Autodesk Inventor part; units mm, degrees
ref_plane "YZ Plane" through (0, 0, 0) normal (1, 0, 0) x (0, 1, 0)
ref_plane "XZ Plane" through (0, 0, 0) normal (0, 1, 0) x (-1, 0, 0)
ref_plane "XY Plane" through (0, 0, 0) normal (0, 0, 1) x (1, 0, 0)
sketch "Skizze1" plane through (0, 0, 0) normal (0, 0, 1) x (1, 0, 0)
  line L0 (0, -42.3366) -> (0, 42.3366) construction
  line L1 (-38.4382, 0) -> (56.3005, 0) construction
  line L2 (0, 0) -> (30.2404, 30.2404) construction
  line L3 (0, 0) -> (42.7664, 0) construction
  line L4 (0, 24.9041) -> (16.9, 24.9041)
  line L5 (16.9, 24.9041) -> (16.9, 21.2841)
  line L6 (16.9, 21.2841) -> (19.092, 19.092)
  line L7 (24.9041, 0) -> (24.9041, 16.9)
  line L8 (24.9041, 16.9) -> (21.2841, 16.9)
  line L9 (21.2841, 16.9) -> (19.092, 19.092)
  line L10 (0, 24.9041) -> (-16.9, 24.9041)
  line L11 (-16.9, 24.9041) -> (-16.9, 21.2841)
  line L12 (-16.9, 21.2841) -> (-19.092, 19.092)
  line L13 (-24.9041, 0) -> (-24.9041, 16.9)
  line L14 (-24.9041, 16.9) -> (-21.2841, 16.9)
  line L15 (-21.2841, 16.9) -> (-19.092, 19.092)
  line L16 (0, 0) -> (30.2404, -30.2404) construction
  line L17 (0, -24.9041) -> (16.9, -24.9041)
  line L18 (16.9, -24.9041) -> (16.9, -21.2841)
  line L19 (16.9, -21.2841) -> (19.092, -19.092)
  line L20 (24.9041, 0) -> (24.9041, -16.9)
  line L21 (24.9041, -16.9) -> (21.2841, -16.9)
  line L22 (21.2841, -16.9) -> (19.092, -19.092)
  line L23 (0, -24.9041) -> (-16.9, -24.9041)
  line L24 (-16.9, -24.9041) -> (-16.9, -21.2841)
  line L25 (-16.9, -21.2841) -> (-19.092, -19.092)
  line L26 (-24.9041, 0) -> (-24.9041, -16.9)
  line L27 (-24.9041, -16.9) -> (-21.2841, -16.9)
  line L28 (-21.2841, -16.9) -> (-19.092, -19.092)
  circle A0 centre (0, 0) radius 10
  dimension "d0" = 45
  dimension "d1" = 16.9
  dimension "d2" = 3.1
  dimension "d3" = 3.62
  dimension "d4" = 20
extrude "Extrusion1" add sketch "Skizze1" along normal blind 2.5
sketch "Skizze2" plane through (0, 0, 2.5) normal (0, 0, 1) x (1, 0, 0)
  line L0 (17.3243, 16.97) -> (5, 16.97) construction
  line L1 (17.3243, 16.97) -> (17.3243, 14.47) construction
  line L2 (5, 14.47) -> (17.3243, 14.47) construction
  line L3 (5, 16.97) -> (5, 14.47) construction
  line L4 (-5, 16.97) -> (-17.3243, 16.97) construction
  line L5 (-5, 16.97) -> (-5, 14.47) construction
  line L6 (-17.3243, 14.47) -> (-5, 14.47) construction
  line L7 (-17.3243, 16.97) -> (-17.3243, 14.47) construction
  circle A0 centre (0, 0) radius 10 construction
  line L8 (16.9, 24.9041) -> (-16.9, 24.9041) construction
  line L9 (-16.9, 24.9041) -> (-16.9, 21.2841) construction
  line L10 (-16.9, 21.2841) -> (-21.2841, 16.9) construction
  line L11 (-21.2841, 16.9) -> (-24.9041, 16.9) construction
  line L12 (-24.9041, 16.9) -> (-24.9041, -16.9) construction
  line L13 (-24.9041, -16.9) -> (-21.2841, -16.9) construction
  line L14 (-21.2841, -16.9) -> (-16.9, -21.2841) construction
  line L15 (-16.9, -21.2841) -> (-16.9, -24.9041) construction
  line L16 (-16.9, -24.9041) -> (16.9, -24.9041) construction
  line L17 (16.9, -24.9041) -> (16.9, -21.2841) construction
  line L18 (16.9, -21.2841) -> (21.2841, -16.9) construction
  line L19 (21.2841, -16.9) -> (24.9041, -16.9) construction
  line L20 (24.9041, -16.9) -> (24.9041, 16.9) construction
  line L21 (24.9041, 16.9) -> (21.2841, 16.9) construction
  line L22 (21.2841, 16.9) -> (16.9, 21.2841) construction
  line L23 (16.9, 21.2841) -> (16.9, 24.9041) construction
  line L24 (-5, 14.47) -> (5, 14.47) construction
  line L25 (5, 14.47) -> (5, 24.9041) construction
  line L26 (5, 24.9041) -> (-5, 24.9041) construction
  line L27 (-5, 24.9041) -> (-5, 14.47) construction
  line L28 (-16.9, 21.2841) -> (-21.2841, 16.9) construction
  line L29 (-16.9, 21.2841) -> (-24.9041, 21.2841) construction
  line L30 (-24.9041, 21.2841) -> (-24.9041, 14.47) construction
  line L31 (-24.9041, 14.47) -> (-16.9, 14.47) construction
  line L32 (-16.9, 14.47) -> (-16.9, 21.2841) construction
  line L33 (0, -34.8857) -> (0, 34.9857) construction
  line L34 (-24.9041, 16.9) -> (-24.9041, -16.9) construction
  line L35 (17.3243, 16.97) -> (17.3243, 14.47) construction
  line L36 (16.9, 21.2841) -> (21.2841, 16.9) construction
  line L37 (21.2841, 16.9) -> (24.9041, 16.9) construction
  line L38 (16.9, 21.2841) -> (21.2841, 16.9) construction
  line L39 (16.9, 21.2841) -> (24.9041, 21.2841) construction
  line L40 (24.9041, 21.2841) -> (24.9041, 14.47) construction
  line L41 (24.9041, 14.47) -> (16.9, 14.47) construction
  line L42 (16.9, 14.47) -> (16.9, 21.2841) construction
  line L43 (16.8, 14.37) -> (25.0041, 14.37)
  line L44 (25.0041, 14.37) -> (25.0041, 21.3841)
  line L45 (25.0041, 21.3841) -> (16.8, 21.3841)
  line L46 (16.8, 21.3841) -> (16.8, 14.37)
  line L47 (-16.8, 14.37) -> (-25.0041, 14.37)
  line L48 (-25.0041, 14.37) -> (-25.0041, 21.3841)
  line L49 (-25.0041, 21.3841) -> (-16.8, 21.3841)
  line L50 (-16.8, 21.3841) -> (-16.8, 14.37)
  line L51 (16.9, 24.9041) -> (-16.9, 24.9041) construction
  line L52 (-5, 14.47) -> (5, 14.47) construction
  line L53 (5, 14.47) -> (5, 24.9041) construction
  line L54 (5, 24.9041) -> (-5, 24.9041) construction
  line L55 (-5, 24.9041) -> (-5, 14.47) construction
  line L56 (5.1, 25.0041) -> (5.1, 14.37)
  line L57 (5.1, 14.37) -> (-5.1, 14.37)
  line L58 (-5.1, 14.37) -> (-5.1, 25.0041)
  line L59 (-5.1, 25.0041) -> (5.1, 25.0041)
  dimension "d8" = 0.1
  dimension "d9" = 0.1
  dimension "d15" = 10
  dimension "d16" = 0.1
extrude "Extrusion2" cut sketch "Skizze2" against normal through all
sketch "Skizze3" plane through (0, 0, 2.5) normal (0, 0, 1) x (1, 0, 0)
  line L0 (16.8, 21.3841) -> (16.9, 21.3841) construction
  line L1 (16.9, 21.3841) -> (16.9, 24.9041) construction
  line L2 (-5.1, 24.9041) -> (-16.9, 24.9041) construction
  line L3 (16.9, 24.9041) -> (5.1, 24.9041) construction
  line L4 (-16.9, 24.9041) -> (-16.9, 21.3841) construction
  line L5 (-16.9, 21.3841) -> (-16.8, 21.3841) construction
  line L6 (-16.8, 21.3841) -> (-16.8, 14.37) construction
  line L7 (-16.8, 14.37) -> (-24.9041, 14.37) construction
  line L8 (-24.9041, 14.37) -> (-24.9041, -16.9) construction
  line L9 (-24.9041, -16.9) -> (-21.2841, -16.9)
  line L10 (-21.2841, -16.9) -> (-16.9, -21.2841)
  line L11 (-16.9, -21.2841) -> (-16.9, -24.9041)
  line L12 (-16.9, -24.9041) -> (16.9, -24.9041) construction
  line L13 (16.9, -24.9041) -> (16.9, -21.2841)
  line L14 (16.9, -21.2841) -> (21.2841, -16.9)
  line L15 (21.2841, -16.9) -> (24.9041, -16.9)
  line L16 (24.9041, -16.9) -> (24.9041, 14.37) construction
  line L17 (24.9041, 14.37) -> (16.8, 14.37) construction
  line L18 (16.8, 14.37) -> (16.8, 21.3841) construction
  circle A0 centre (0, 0) radius 10 construction
  line L19 (24.8041, -16.8) -> (21.2426, -16.8)
  line L20 (21.2426, -16.8) -> (16.8, -21.2426)
  line L21 (16.8, -21.2426) -> (16.8, -24.8041)
  line L22 (16.8, -24.8041) -> (-16.8, -24.8041) construction
  line L23 (-16.8, -24.8041) -> (-16.8, -21.2426)
  line L24 (-16.8, -21.2426) -> (-21.2426, -16.8)
  line L25 (-21.2426, -16.8) -> (-24.8041, -16.8)
  line L26 (-24.8041, -16.8) -> (-24.8041, 14.27) construction
  line L27 (-24.8041, 14.27) -> (-16.7, 14.27) construction
  line L28 (-16.7, 14.27) -> (-16.7, 21.4841) construction
  line L29 (-16.7, 21.4841) -> (-16.8, 21.4841) construction
  line L30 (-16.8, 21.4841) -> (-16.8, 24.8041) construction
  line L31 (-16.8, 24.8041) -> (-2.7, 24.8041) construction
  line L32 (-2.7, 24.8041) -> (-2.7, 14.27) construction
  line L33 (-2.7, 14.27) -> (2.7, 14.27) construction
  line L34 (2.7, 14.27) -> (2.7, 24.8041) construction
  line L35 (2.7, 24.8041) -> (16.8, 24.8041) construction
  line L36 (16.8, 24.8041) -> (16.8, 21.4841) construction
  line L37 (16.8, 21.4841) -> (16.7, 21.4841) construction
  line L38 (16.7, 21.4841) -> (16.7, 14.27) construction
  line L39 (16.7, 14.27) -> (24.8041, 14.27) construction
  line L40 (24.8041, 14.27) -> (24.8041, -16.8) construction
  line L41 (-24.8041, -16.8) -> (-24.8041, -16.9)
  line L42 (-16.8, -24.8041) -> (-16.9, -24.8041)
  line L43 (16.8, -24.8041) -> (16.9, -24.8041)
  line L44 (24.8041, -16.8) -> (24.8041, -16.9)
  line L45 (5.1, 24.9041) -> (5.1, 14.37)
  line L46 (5.1, 14.37) -> (-5.1, 14.37)
  line L47 (-5.1, 14.37) -> (-5.1, 24.9041)
  dimension "d12" = 0.1
extrude "Extrusion3" cut sketch "Skizze3" against normal up to surface (2.5 mm away)
mirror "Spiegeln1" about plane through (0, 0, 0) normal (0, 1, 0) of "Extrusion2"
ref_plane "Arbeitsebene1" through (0, 0, 1.25) normal (0, 0, 1) x (1, 0, 0)
sketch "Skizze4" plane through (0, 0, 2.5) normal (0, 0, 1) x (1, 0, 0)
  circle A0 centre (0, 0) radius 10 construction
  line L0 (-24.9041, -14.37) -> (-16.8, -14.37) construction
  line L1 (-16.8, -14.37) -> (-16.8, -24.8041) construction
  line L2 (-16.8, -24.8041) -> (-16.9, -24.8041) construction
  line L3 (-16.9, -24.8041) -> (-16.9, -24.9041) construction
  line L4 (-16.9, -24.9041) -> (-5.1, -24.9041) construction
  line L5 (-5.1, -24.9041) -> (-5.1, -14.37) construction
  line L6 (-5.1, -14.37) -> (5.1, -14.37) construction
  line L7 (5.1, -14.37) -> (5.1, -24.9041) construction
  line L8 (5.1, -24.9041) -> (16.9, -24.9041) construction
  line L9 (16.9, -24.9041) -> (16.9, -24.8041) construction
  line L10 (16.9, -24.8041) -> (16.8, -24.8041) construction
  line L11 (16.8, -24.8041) -> (16.8, -14.37) construction
  line L12 (16.8, -14.37) -> (24.9041, -14.37) construction
  line L13 (24.9041, -14.37) -> (24.9041, 14.37) construction
  line L14 (24.9041, 14.37) -> (16.8, 14.37) construction
  line L15 (16.8, 14.37) -> (16.8, 21.3841) construction
  line L16 (16.8, 21.3841) -> (16.9, 21.3841) construction
  line L17 (16.9, 21.3841) -> (16.9, 24.9041) construction
  line L18 (16.9, 24.9041) -> (5.1, 24.9041) construction
  line L19 (5.1, 24.9041) -> (5.1, 14.37) construction
  line L20 (5.1, 14.37) -> (-5.1, 14.37) construction
  line L21 (-5.1, 14.37) -> (-5.1, 24.9041) construction
  line L22 (-5.1, 24.9041) -> (-16.9, 24.9041) construction
  line L23 (-16.9, 24.9041) -> (-16.9, 21.3841) construction
  line L24 (-16.9, 21.3841) -> (-16.8, 21.3841) construction
  line L25 (-16.8, 21.3841) -> (-16.8, 14.37) construction
  line L26 (-16.8, 14.37) -> (-24.9041, 14.37) construction
  line L27 (-24.9041, 14.37) -> (-24.9041, -14.37) construction
  line L28 (5.1, 24.9041) -> (3.6, 24.9041)
  line L29 (3.6, 24.9041) -> (3.6, 22.4041)
  line L30 (3.6, 22.4041) -> (5.1, 22.4041)
  line L31 (5.1, 22.4041) -> (5.1, 24.9041)
  line L32 (-34.8657, 0) -> (34.8657, 0) construction
  line L33 (0, 34.8657) -> (0, -34.8657) construction
  line L34 (5.1, -24.9041) -> (3.6, -24.9041)
  line L35 (3.6, -24.9041) -> (3.6, -22.4041)
  line L36 (3.6, -22.4041) -> (5.1, -22.4041)
  line L37 (5.1, -22.4041) -> (5.1, -24.9041)
  line L38 (-5.1, 24.9041) -> (-3.6, 24.9041)
  line L39 (-3.6, 24.9041) -> (-3.6, 22.4041)
  line L40 (-3.6, 22.4041) -> (-5.1, 22.4041)
  line L41 (-5.1, 22.4041) -> (-5.1, 24.9041)
  line L42 (-3.6, -22.4041) -> (-5.1, -22.4041)
  line L43 (-3.6, -24.9041) -> (-3.6, -22.4041)
  line L44 (-5.1, -24.9041) -> (-3.6, -24.9041)
  line L45 (-5.1, -22.4041) -> (-5.1, -24.9041)
  dimension "d18" = 2.5
  dimension "d19" = 1.5
extrude "Extrusion4" add sketch "Skizze4" against normal up to surface (2.5 mm away)
sketch "Skizze5" plane through (3.6, 22.4041, 2.5) normal (-1, 0, 0) x (0, 0, 1)
  line L0 (-2.5, 0) -> (-2.5, 2.5) construction
  line L1 (0, 0) -> (-2.5, 0) construction
  line L2 (0, 2.5) -> (0, 0) construction
  line L3 (0, 2.5) -> (-2.5, 2.5) construction
  circle A0 centre (-1.25, 1.25) radius 1.25
  line L4 (-1.25, 12.4616) -> (-1.25, -57.2697)
  line L5 (0, 2.5) -> (-2.5, 2.5)
  line L6 (-2.5, 2.5) -> (-2.5, 0)
  line L7 (-2.5, 0) -> (0, 0)
  line L8 (0, 0) -> (0, 2.5)
  point P0 (-2.5, -22.4041)
extrude "Extrusion5" cut sketch "Skizze5" against normal up to surface (1.5 mm away) contours L8 L7 A0 | A0 L5 L8 | A0 L6 L5 | L7 L6 A0
mirror "Spiegeln2" about plane through (0, 0, 0) normal (0, 1, 0) of "Extrusion5"
mirror "Spiegeln3" about plane through (0, 0, 0) normal (1, 0, 0) of "Extrusion5", "Spiegeln2"
properties part number "20_Cube_Insert_focusing_holder_v3"
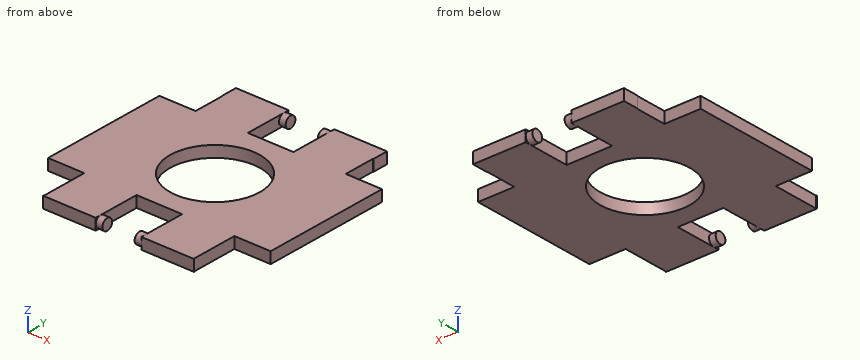
Verification items for the finished model (mm, model axes). Give positions to 0.01 mm unless a question says otherwise; leave off trailing zeros. Order: outer loops, then holes, each group sorted by start corner. A loop starts at its lowest first (then second) coordinate and runs counter-clockwise, first axis right, second up. Notation, with made-up numbers: M 10,66.25 L 59,66.25 A14 cw 59,91.25 Z; hole C 12.25,54 d4. An arc over 180 degrees is marked long. Answer as a JSON object with one key per item and string values. Group by question number.
1) Scan lines: line 1 along Y through (x, z) = (0, 0.7); line 2 along X through (y, z) = (-20, 2); line 3 along X through (y, z) = (21.5, 1). Record each from-to range of solid material in increasing order. Write a range as [from, to].
2) Cross-section at A-A (y = 0). Enter the section's corners in (x, z).
3) Cross-section at B-B (x = 0.5). Enter the section's corners in (y, z), then the cut area to 3 significant figures.
4) Depth check by flat-ended pin: pin 1 Ø1.2 at (y, z) = (24, 1.5) entering from -X; pin 2 Ø1 at (y, z) = (-24, 1) entering from -X; pin 3 Ø1.2 at (x, z) = (1.5, 1.5) entering from -Y. Enter the tip coordinate at first touch or a pass-through.
Result sheet:
{
 "1": {"line 1": "y = [-14.37, -10], [10, 14.37]", "line 2": "x = [-16.8, -5.1], [5.1, 16.8]", "line 3": "x = [-16.9, -5.1], [5.1, 16.9]"},
 "2": {"outline": "M -24.9,0 L -10,0 L -10,2.5 L -24.9,2.5 Z; M 10,0 L 24.9,0 L 24.9,2.5 L 10,2.5 Z"},
 "3": {"outline": "M -14.37,0 L -9.99,0 L -9.99,2.5 L -14.37,2.5 Z; M 9.99,0 L 14.37,0 L 14.37,2.5 L 9.99,2.5 Z", "area": "21.9 mm2"},
 "4": {"pin 1": "stops at x = -16.9", "pin 2": "stops at x = -16.8", "pin 3": "stops at y = -14.37"}
}
